Can you work these out from the model? Positions are in its coordinate system, mm. A direction names the side the tool comes from. Give positions to 0.01 mm unless a question says otherwise; leave off trailing zeros. Order: outer loops, then holes, each group sorted by start corner. A loop starts at its lowest first (then second) coordinate and runs counter-clockwise, first axis right, second up. Notation, with made-up numbers: (-1, -29) -> (30, -29) arc R20 ccw to (30, -9) -> close; hole circle Ø10 at (-15.75, -4). An arc over 180 degrees is marked (long way). Answer as CSV lines item,"result".
Autodesk Inventor part; units mm, degrees
ref_plane "YZ Plane" through (0, 0, 0) normal (1, 0, 0) x (0, 1, 0)
ref_plane "XZ Plane" through (0, 0, 0) normal (0, 1, 0) x (-1, 0, 0)
ref_plane "XY Plane" through (0, 0, 0) normal (0, 0, 1) x (1, 0, 0)
sketch "Sketch1" plane through (0, 0, 0) normal (0, 0, 1) x (1, 0, 0)
  line L0 (0, 0) -> (49.8, 0)
  line L1 (49.8, 0) -> (49.8, 36.921)
  line L2 (49.8, 36.921) -> (0, 36.921)
  line L3 (0, 36.921) -> (0, 0)
  dimension "d0" = 49.8
  dimension "d1" = 36.921
extrude "Extrusion1" add sketch "Sketch1" along normal blind 5
sketch "Sketch2" plane through (0, 0, 0) normal (0, 0, -1) x (-1, 0, 0)
  line L0 (0, 0) -> (-49.8, 0)
  line L1 (0, 0) -> (-49.8, 0)
  line L2 (-49.8, 0) -> (-49.8, 5)
  line L3 (-49.8, 5) -> (0, 5)
  line L4 (0, 5) -> (0, 0)
  dimension "d4" = 49.8
  dimension "d5" = 5
extrude "Extrusion2" add sketch "Sketch2" along normal blind 30
sketch "Sketch4" plane through (0, 0, 0) normal (0, 0, -1) x (-1, 0, 0)
  line L0 (-38.9, 36.921) -> (-10.9, 36.921)
  line L1 (-10.9, 36.921) -> (-10.9, 12)
  line L2 (-10.9, 12) -> (-38.9, 12)
  line L3 (-38.9, 12) -> (-38.9, 36.921)
  line L4 (0, 36.921) -> (0, 5)
  line L5 (0, 5) -> (-49.8, 5)
  point P0 (0, 0)
  dimension "d24" = 28
  dimension "d25" = 24.921
  dimension "d26" = 10.9
  dimension "d27" = 7
extrude "Extrusion3" cut sketch "Sketch4" against normal through all
sketch "Sketch6" plane through (0, 5, 0) normal (0, 1, 0) x (1, 0, 0)
  line L0 (0, -32.5) -> (49.8, -32.5)
  line L1 (49.8, -32.5) -> (49.8, 17.3)
  line L2 (49.8, 17.3) -> (0, 17.3)
  line L3 (0, 17.3) -> (0, -32.5)
  circle A0 centre (44.9, 9.4) radius 1.45
  circle A1 centre (4.9, 9.4) radius 1.45
  line L4 (24.9, 17.3) -> (24.9, 7.3)
  circle A2 centre (45.7, 3.9) radius 2.55
  circle A3 centre (39.4, 10.2) radius 2.55
  circle A4 centre (4.1, 3.9) radius 2.55
  circle A5 centre (10.4, 10.2) radius 2.55
  line L5 (49.8, 0) -> (49.8, 30)
  line L6 (0, 17.3) -> (49.8, 17.3)
  line L7 (49.8, 17.3) -> (49.8, 30)
  line L8 (49.8, 30) -> (0, 30)
  line L9 (0, 30) -> (0, 17.3)
  line L10 (49.8, 30) -> (49.8, -5)
  line L11 (0, 17.3) -> (49.8, 17.3)
  line L12 (49.8, 17.3) -> (49.8, 14.3)
  line L13 (49.8, 14.3) -> (0, 14.3)
  line L14 (0, 14.3) -> (0, 17.3)
  point P0 (0, 0)
  dimension "d36" = 49.8
  dimension "d37" = 49.8
  dimension "d38" = 2.9
  dimension "d39" = 4.9
  dimension "d40" = 7.9
  dimension "d41" = 2.9
  dimension "d42" = 4.9
  dimension "d43" = 7.9
  dimension "d44" = 10
  dimension "d45" = 5.1
  dimension "d46" = 5.1
  dimension "d47" = 4.1
  dimension "d48" = 13.4
  dimension "d49" = 10.4
  dimension "d50" = 7.1
  dimension "d64" = 3
extrude "Extrusion5" cut sketch "Sketch6" against normal through all contours L3 L2 L4 L13 | L9 L8 L5 L2 | L4 L2 L1 L13 | A0 | A1 | A2 | A3 | A4 | A5
sketch "Sketch8" plane through (0, 0, 5) normal (0, 0, 1) x (1, 0, 0)
  line L0 (0, 0) -> (49.8, 0)
  line L1 (0, 0) -> (49.8, 0)
  line L2 (49.8, 0) -> (49.8, 2.5)
  line L3 (49.8, 2.5) -> (0, 2.5)
  line L4 (0, 2.5) -> (0, 0)
  dimension "d53" = 2.5
extrude "Extrusion6" add sketch "Sketch8" along normal blind 12.7
sketch "Sketch9" plane through (0, 2.5, 5) normal (0, 1, 0) x (1, 0, 0)
  circle A0 centre (44.9, -7.8) radius 1.45
  circle A1 centre (4.9, -7.8) radius 1.45
  line L0 (0, 0) -> (0, -12.7)
  line L1 (49.8, -12.7) -> (0, -12.7)
  line L2 (49.8, 0) -> (49.8, -12.7)
  point P0 (0, 5)
  dimension "d56" = 2.9
  dimension "d57" = 2.9
  dimension "d58" = 4.9
  dimension "d59" = 4.9
  dimension "d60" = 4.9
  dimension "d61" = 4.9
extrude "Extrusion7" cut sketch "Sketch9" against normal through all
fillet "Fillet1" radius 2 2 edges at (49.8, 2.5, -14.3) (0, 2.5, -14.3)
sketch "Sketch10" plane through (0, 0, 0) normal (0, 0, -1) x (-1, 0, 0)
  line L0 (-10.9, 36.921) -> (-10.9, 12)
  line L1 (-10.9, 12) -> (-38.9, 12)
  line L2 (-38.9, 12) -> (-38.9, 36.921)
  line L3 (-49.8, 36.921) -> (-38.9, 36.921)
  line L4 (-49.8, 5) -> (-49.8, 36.921)
  line L5 (-49.8, 5) -> (0, 5)
  line L6 (0, 36.921) -> (0, 5)
  line L7 (-10.9, 36.921) -> (0, 36.921)
  line L8 (-10.9, 18.4272) -> (-10.9, 27.6034)
  point P0 (0, 0)
extrude "Extrusion8" add sketch "Sketch10" along normal blind 5
sketch "Sketch3" plane through (0, 0, 0) normal (0, 0, -1) x (-1, 0, 0)
  circle A0 centre (-44.9, 31.921) radius 1.4
  circle A1 centre (-4.9, 31.921) radius 1.4
  circle A2 centre (-4.9, 12) radius 1.4
  line L0 (-49.8, 5) -> (-49.8, 36.921)
  line L1 (-49.8, 36.921) -> (0, 36.921)
  line L2 (0, 36.921) -> (0, 5)
  line L3 (0, 5) -> (-49.8, 5)
  circle A3 centre (-44.9, 12) radius 1.4
  point P0 (0, 0)
  dimension "d8" = 2.8
  dimension "d9" = 2.8
  dimension "d10" = 2.8
  dimension "d11" = 4.9
  dimension "d12" = 5
  dimension "d13" = 5
  dimension "d14" = 4.9
  dimension "d15" = 4.9
  dimension "d16" = 7
  dimension "d30" = 2.8
  dimension "d31" = 4.9
  dimension "d32" = 7
extrude "Extrusion9" cut sketch "Sketch3" against normal blind 5 and the other way blind 5 contours A0 | A1 | A2 | A3
sketch "Sketch11" plane through (0, 0, -5) normal (0, 0, -1) x (-1, 0, 0)
  circle A0 centre (-44.9, 31.921) radius 1.4
  circle A1 centre (-44.9, 31.921) radius 3
  circle A2 centre (-44.9, 12) radius 1.4
  circle A3 centre (-44.9, 12) radius 3
  circle A4 centre (-4.9, 31.921) radius 1.4
  circle A5 centre (-4.9, 31.921) radius 3
  circle A6 centre (-4.9, 12) radius 1.4
  circle A7 centre (-4.9, 12) radius 3
  point P0 (0, 0)
  dimension "d72" = 6
  dimension "d73" = 6
  dimension "d74" = 6
  dimension "d75" = 6
extrude "Extrusion10" cut sketch "Sketch11" against normal blind 2
sketch "Sketch12" plane through (0, 0, 5) normal (0, 0, 1) x (1, 0, 0)
  line L0 (38.9, 12) -> (10.9, 12)
  line L1 (13, 12) -> (36.9, 12)
  line L2 (36.9, 12) -> (36.9, 6)
  line L3 (36.9, 6) -> (13, 6)
  line L4 (13, 6) -> (13, 12)
  point P0 (0, 0)
  dimension "d78" = 23.9
  dimension "d79" = 6
extrude "Extrusion11" cut sketch "Sketch12" against normal blind 10
fillet "Fillet2" radius 2 2 edges at (13, 12, 0) (36.9, 12, 0)
properties part number "30_CUBE_openSIM_DMD_Fixation_base"
Item 1: Imagine slicing it at A-A, the plane y = 20. Please give me the cut outline in (x, z).
Numbers:
outline,"(0, -5) -> (10.9, -5) -> (10.9, 5) -> (0, 5) -> close; (38.9, -5) -> (49.8, -5) -> (49.8, 5) -> (38.9, 5) -> close"
Item 2: For pin 1 (6.5 mm diameter, centred on x = 5, y = 32.5, fed in from -Z); pin 2 (5.5 mm diameter, centred on x = 44.9, y = 31.921, fed in from -Z); pin 3 (7.5 mm diameter, centred on x = 25, z = -9.5, fed in from +Y), each with a flat end and sliding along its axis, tell me the tip position at first contact or that it passes through.
Numbers:
pin 1,"stops at z = -5"
pin 2,"stops at z = -3"
pin 3,"stops at y = 5"
Item 3: For faces 5 (the flat face through (13, 8, 0)), 6 (the cylindrical face through (48, 3, -5)), 7 (the flat face through (42, 21, -5)), 8 (the cylindrical face through (43.287, 34.451, -4.014)), 9 (the flat face through (25, 2.5, 11)), which set-ups out of +Z, -Z, +X, -X, +Y, -Y let a thin tool reach every point of the face, with its end or its side?
Numbers:
face 5,"+Z, -Z, +Y"
face 6,"-Y"
face 7,"-Z, +X, -X, +Y"
face 8,"-Z"
face 9,"+Z, +X, -X, +Y"
Item 4: Imagine slicing it at B-B, the plane z = -10.2. Please give me the cut outline in (x, y), then the cut area to 3 significant figures.
Numbers:
outline,"(0, 0) -> (3.69, 0) -> (3.69, 5) -> (0, 5) -> close; (6.11, 0) -> (7.85, 0) -> (7.85, 5) -> (6.11, 5) -> close; (12.95, 0) -> (36.85, 0) -> (36.85, 5) -> (12.95, 5) -> close; (41.95, 0) -> (43.69, 0) -> (43.69, 5) -> (41.95, 5) -> close; (46.11, 0) -> (49.8, 0) -> (49.8, 5) -> (46.11, 5) -> close"
area,"174 mm²"
Item 5: We'd pull the mould along Y, two halves only. Please class faces 1 (the cylindrical face through (3.287, 34.451, -4.014)), 2 (the cylindrical face through (6.01, 31.07, 0.94)), 3 (the flat face through (25, 1, 17.7)), 4 (the flat face through (25, 5, -10)): released by +Y, released by -Y, zero draft, split by the parting line, or undercut.
Numbers:
face 1,"undercut"
face 2,"undercut"
face 3,"zero draft"
face 4,"released by +Y"
Item 6: Imagine slicing it at C-C, the plane x = 34. Please give me the cut outline in (y, z), then the cut area to 3 significant figures.
Numbers:
outline,"(0, -14.3) -> (5, -14.3) -> (5, -5) -> (6, -5) -> (6, 5) -> (2.5, 5) -> (2.5, 17.7) -> (0, 17.7) -> close"
area,"138 mm²"
Item 7: Imagine slicing it at D-D, the plane z = 0. Give the number of separate pieces and of enclosed holes in the cut face, then the cut area to 3 significant figures.
Numbers:
separate pieces,"1"
enclosed holes,"4"
area,"971 mm²"
Item 8: Please list where these lines run through material, in increasing order: line 1 along Y through (x, z) = (44.9, 1.5); line 2 along Y through (x, z) = (5.5, -3.5); line 3 along X through (y, z) = (3, -10.5).
Numbers:
line 1,"y = 0 to 10.6, 13.4 to 30.52, 33.32 to 36.92"
line 2,"y = 5 to 9.06, 14.94 to 28.98, 34.86 to 36.92"
line 3,"x = 0 to 3.96, 5.84 to 7.87, 12.93 to 36.87, 41.93 to 43.96, 45.84 to 49.8"
